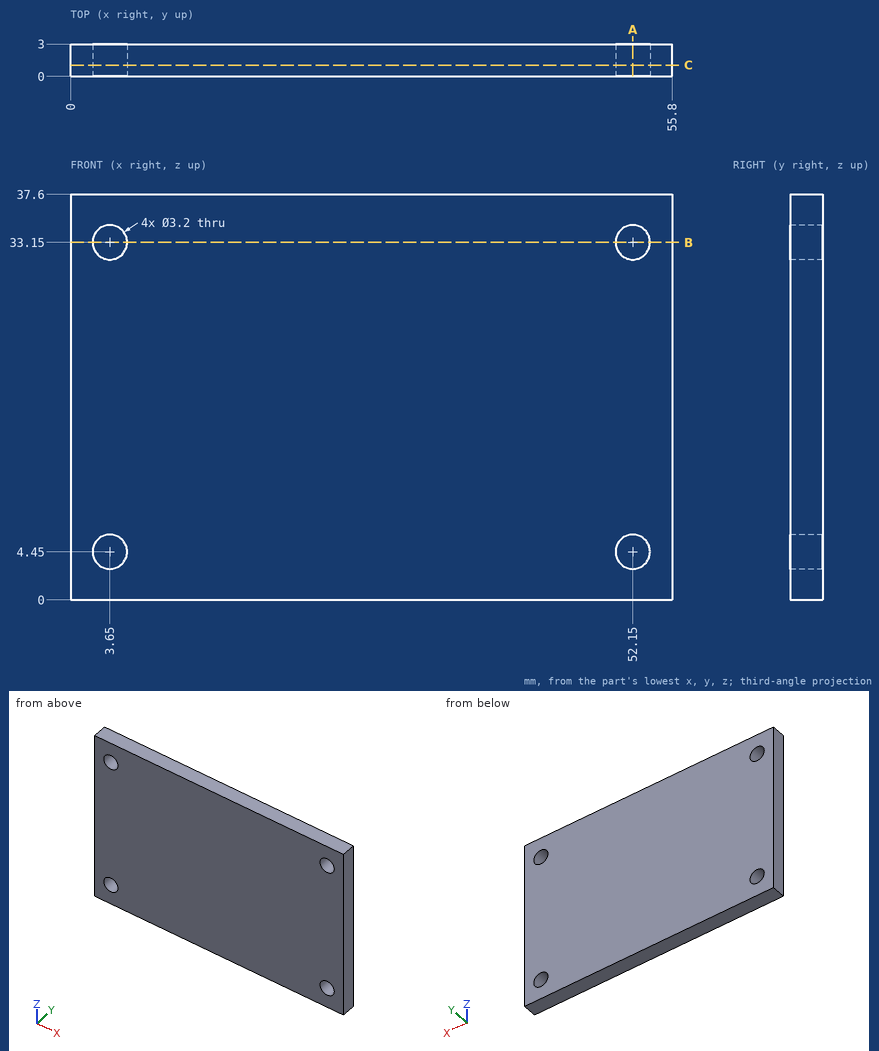
Geometry: see drawing. Coordinates: mm, zero at the bounding-box minimum. Give positions to 0.01 mm unless a question says otherwise; leave off trailing zeros. Order: outer loops, then holes, each group sorted by start corner. A loop starts at its lowest first (then second) coordinate and runs counter-clockwise, first axis right, second up. Notation, with made-up numbers: (18.5, -2.5) - (63.5, -2.5) arc R32 ccw to (63.5, 34.5) - close; hole circle Ø8 at (7, 86.25). An arc over 180 degrees is marked (long way). One line per item, written item: value.
1. Cut plane A-A, the plane x = 52.15. Output: boundary loops of the cut face in (y, z), and give its area (3 significant figures).
Determined:
outline: (0, 0) - (3, 0) - (3, 2.85) - (0, 2.85) - close; (0, 6.05) - (3, 6.05) - (3, 31.55) - (0, 31.55) - close; (0, 34.75) - (3, 34.75) - (3, 37.6) - (0, 37.6) - close
area: 93.6 mm2
2. Line query: probe 1 along Z at (x, y) = (52.15, 1.85); probe 2 along X at (y, z) = (1.6, 33.15); probe 3 along X at (y, z) = (2.55, 32). Output: solid intervals per line, ascending.
Determined:
probe 1: 0 to 2.85, 6.05 to 31.55, 34.75 to 37.6
probe 2: 0 to 2.05, 5.25 to 50.55, 53.75 to 55.8
probe 3: 0 to 2.54, 4.76 to 51.04, 53.26 to 55.8
3. Cut plane B-B, the plane z = 33.15. Output: boundary loops of the cut face in (x, y), and give its area (3 significant figures).
Determined:
outline: (0, 0) - (2.05, 0) - (2.05, 3) - (0, 3) - close; (5.25, 0) - (50.55, 0) - (50.55, 3) - (5.25, 3) - close; (53.75, 0) - (55.8, 0) - (55.8, 3) - (53.75, 3) - close
area: 148 mm2
4. Cut plane C-C, the plane y = 1.05. Output: boundary loops of the cut face in (x, z), and give its area (3 significant figures).
Determined:
outline: (0, 0) - (55.8, 0) - (55.8, 37.6) - (0, 37.6) - close; hole circle Ø3.2 at (3.65, 4.45); hole circle Ø3.2 at (3.65, 33.15); hole circle Ø3.2 at (52.15, 4.45); hole circle Ø3.2 at (52.15, 33.15)
area: 2,070 mm2
5. Pin query (flat end, axial travel): pin 1 Ø2.5 at (x, z) = (3.65, 4.45) entering from -Y. Return the tip coordinate at first contact, or that it passes through.
Determined:
pin 1: through
